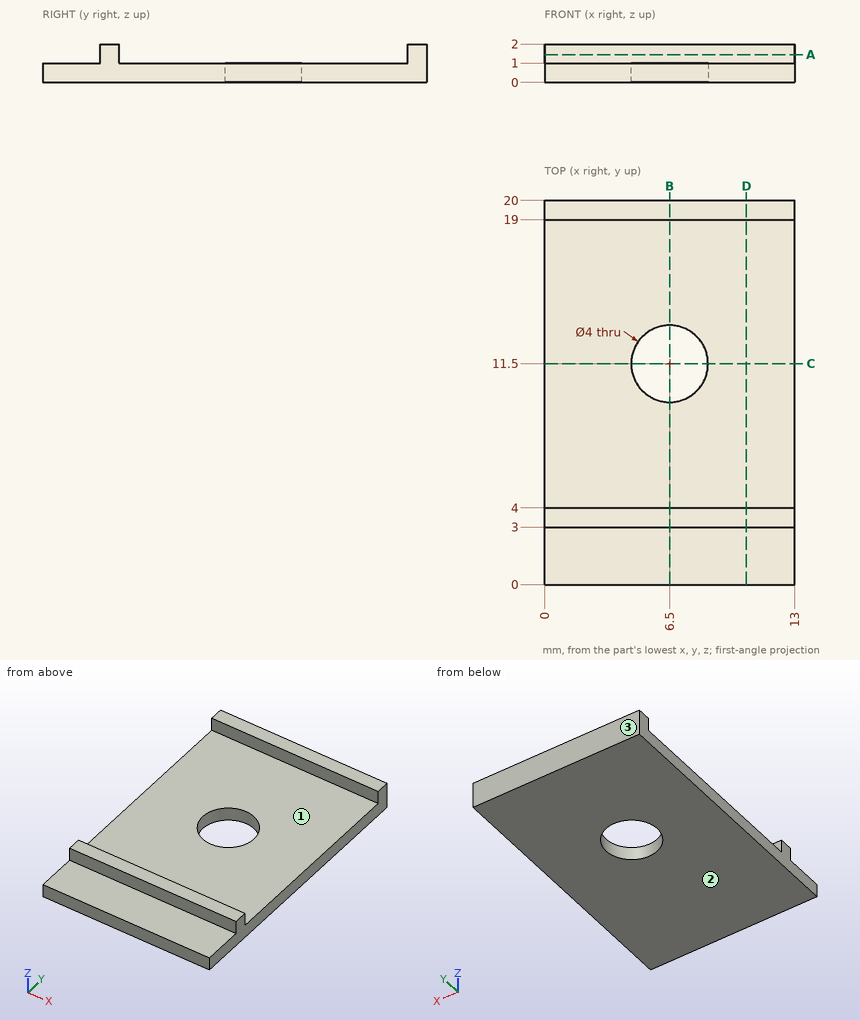
The figure shows three views and two pictorial views of one solid part (mm, origin at its lowest corner). Answer the questions. Give positions to 0.01 mm unless a question says otherwise; leave off trailing zeros. Write each loop counter-clockwise with the first axis right and the second up, starting at its lowest first coordinate (ties: lowest second). Pieces come first, ordered by that corner, then holes. Notation, with made-up numbers: (-5.5, 2.25) -> (46.5, 2.25) arc R28 cw to (46.5, 23.25) -> close; hole circle Ø10 at (-11.75, 0.25). An arc over 180 degrees is marked (long way). Use one line per item in the form item = value.
1) For a pull along Y with two mould halves and no side action, classify the marked faces 1, 2 and 3 as +Y half, -Y half, draft (parallel to the pull), parting line (faces both ways), or undercut.
Result:
face_1 = undercut
face_2 = draft
face_3 = +Y half
2) Each of these flat-tipped pins is pushed along its axis until it touches: P1, Ø6, axis at x = 9, y = 12, coming from the +Z side; P2, Ø0.5, axis at x = 7, z = 1.5, coming from the -Y side. Where does it stop, or does it pass through?
Result:
P1 = 1
P2 = 3
3) Section D-D on x = 10.5 is taken. Write down the section's boundary in (y, z), plus the area to 3 significant figures.
Result:
outline = (0, 0) -> (20, 0) -> (20, 2) -> (19, 2) -> (19, 1) -> (4, 1) -> (4, 2) -> (3, 2) -> (3, 1) -> (0, 1) -> close
area = 22.0 mm²
4) Section A-A on z = 1.45 is taken. Write down the section's boundary in (x, y).
Result:
outline = (0, 3) -> (13, 3) -> (13, 4) -> (0, 4) -> close; (0, 19) -> (13, 19) -> (13, 20) -> (0, 20) -> close
5) Straight lines are drawn through the part: probe 1 along Y at (x, z) = (6.5, 0.5); probe 2 along Y at (x, z) = (9.5, 1.75); probe 3 along Z at (x, y) = (4.75, 5). For each, find the intervals that lie inside material, in ascending order.
Result:
probe_1 = 0 to 9.5, 13.5 to 20
probe_2 = 3 to 4, 19 to 20
probe_3 = 0 to 1
6) Section C-C on y = 11.5 is taken. Write down the section's boundary in (x, z).
Result:
outline = (0, 0) -> (4.5, 0) -> (4.5, 1) -> (0, 1) -> close; (8.5, 0) -> (13, 0) -> (13, 1) -> (8.5, 1) -> close
7) Section B-B on x = 6.5 is taken. Write down the section's boundary in (y, z), plus the area to 3 significant figures.
Result:
outline = (0, 0) -> (9.5, 0) -> (9.5, 1) -> (4, 1) -> (4, 2) -> (3, 2) -> (3, 1) -> (0, 1) -> close; (13.5, 0) -> (20, 0) -> (20, 2) -> (19, 2) -> (19, 1) -> (13.5, 1) -> close
area = 18.0 mm²
